Verification items for the finished model (mm, model axes). A direction names the side the tool comes from. Give positions to 0.01 mm unless a question says otherwise; leave off trailing zeros. Write each loop counter-clockwise with the first axis right and the second up, starting at its lowest first coordinate (ties: lowest second). Pieces come first, ordered by that corner, then holes. Notation, with made-up numbers: (79.5, 20.25) - (134.5, 20.25) arc R20 cw to (134.5, 49.25) - close; hole circle Ø11 at (32.5, 61.25). An arc over 180 degrees is marked (long way). Answer as a JSON object with one key per item and string values. Group by question number.
Item 1: Tool access check on faces 1 (the face through (3.176, -567, 9)), 2 (the face through (600, -53, 9)), 3 (the face through (611, -415, 9)), 4 (the face through (295, -53.941, 9)), 5 (the face through (-9, -205, 9)). Record the directions out of +Z, -Z, +X, -X, +Y, -Y that give a thin tool (end or side, any length) a straight path to the whole face; none if there is none.
Item 2: Go/stop test with flat-tipped pins: pin 1 (9 mm diameter, centred on y = -551, z = 4.5, fed in from +X); pin 2 (9 mm diameter, centred on y = -560.5, z = 7.5, fed in from -X); pin 3 (5.5 mm diameter, centred on y = -511, z = 12, fed in from -X). Record where each tip stops, or that it passes through.
Item 3: Sectioned sample at A-A, the plane z = 5. Record the boundary of the cut face in (x, y).
Item 4: Scan lines: line 1 along X through (y, z) = (-485.5, 8.25); line 2 along X through (y, z) = (-110, 2); line 3 along X through (y, z) = (-437.5, 11). Record each from-to range of solid material in increasing order. Write a range as [from, to].
Item 5: Sectioned sample at C-C, the plane y = -437.5. Record the boundary of the cut face in (x, z), and give its area (3 significant figures).
Item 6: Sectioned sample at B-B, the plane y = -371.5. Record the boundary of the cut face in (x, z), and give its area (3 significant figures).
Item 7: Draft check along Y on faces 6 (the face through (276.972, -517, 9)), 7 (the face through (-6.78, -464, 9)), 8 (the face through (612, -515, 9)). Enter one of: +Y half, -Y half, draft (parallel to the pull), parting line (faces both ways), or undercut.
```python
from build123d import *

# Parameters (mm, degrees)
BOSS_EXTRUDE3_DEPTH     = 18
CUT_EXTRUDE1_DEPTH      = 878.82331891
CUT_EXTRUDE1_DEPTH_BACK = 878.82331891
SKETCH2_W               = 36
SKETCH2_H               = 100


with BuildPart() as part:
    # Sketch1 → Boss-Extrude3 (new body)
    with BuildSketch(Plane.XY):
        Polygon((0, 0), (0, -105), (-18, -105), (-18, -205), (0, -205), (0, -415), (-6.780081157, -415), (-6.780081157, -515), (3.176196781, -514.99186428), (3.176196781, -619.99186428), (603.176196781, -619.99186428), (603.176196781, -515), (621.176196781, -515), (621.176196781, -415), (600, -415), (600, -205), (621.176196781, -205), (621.176196781, -105), (600, -105), (600, 0), align=None)
    extrude(amount=BOSS_EXTRUDE3_DEPTH)

    # Sketch2 → Cut-Extrude1 (cut, two sides: drawn at the far end of the back side and taken through both)
    with BuildSketch(Plane(origin=(0, 0, 0), x_dir=(-1, 0, 0), z_dir=(0, 0, -1)).offset(-CUT_EXTRUDE1_DEPTH_BACK)):
        with Locations((-294.972181327, -103.940998789)):
            Rectangle(SKETCH2_W, SKETCH2_H)
        with Locations((-294.972181327, -516.059001211)):
            Rectangle(SKETCH2_W, SKETCH2_H)
    extrude(amount=CUT_EXTRUDE1_DEPTH + CUT_EXTRUDE1_DEPTH_BACK, mode=Mode.SUBTRACT)


solid = part.part
```
Geometry check:
{
 "1": {"face 1": "+Z, -Z, -X, -Y", "face 2": "+Z, -Z, +X, +Y", "face 3": "+Z, -Z, +X", "face 4": "+Z, -Z", "face 5": "+Z, -Z, -X"},
 "2": {"pin 1": "x = 603.18", "pin 2": "x = 3.18", "pin 3": "x = -6.78"},
 "3": {"outline": "(-18, -205) - (0, -205) - (0, -415) - (-6.78, -415) - (-6.78, -515) - (3.18, -514.99) - (3.18, -619.99) - (603.18, -619.99) - (603.18, -515) - (621.18, -515) - (621.18, -415) - (600, -415) - (600, -205) - (621.18, -205) - (621.18, -105) - (600, -105) - (600, 0) - (0, 0) - (0, -105) - (-18, -105) - close; hole (276.97, -566.06) - (312.97, -566.06) - (312.97, -466.06) - (276.97, -466.06) - close; hole (276.97, -153.94) - (312.97, -153.94) - (312.97, -53.94) - (276.97, -53.94) - close"},
 "4": {"line 1": "[-6.78, 276.97], [312.97, 621.18]", "line 2": "[-18, 276.97], [312.97, 621.18]", "line 3": "[-6.78, 621.18]"},
 "5": {"outline": "(-6.78, 0) - (621.18, 0) - (621.18, 18) - (-6.78, 18) - close", "area": "11,300 mm^2"},
 "6": {"outline": "(0, 0) - (600, 0) - (600, 18) - (0, 18) - close", "area": "10,800 mm^2"},
 "7": {"face 6": "undercut", "face 7": "draft", "face 8": "-Y half"}
}
